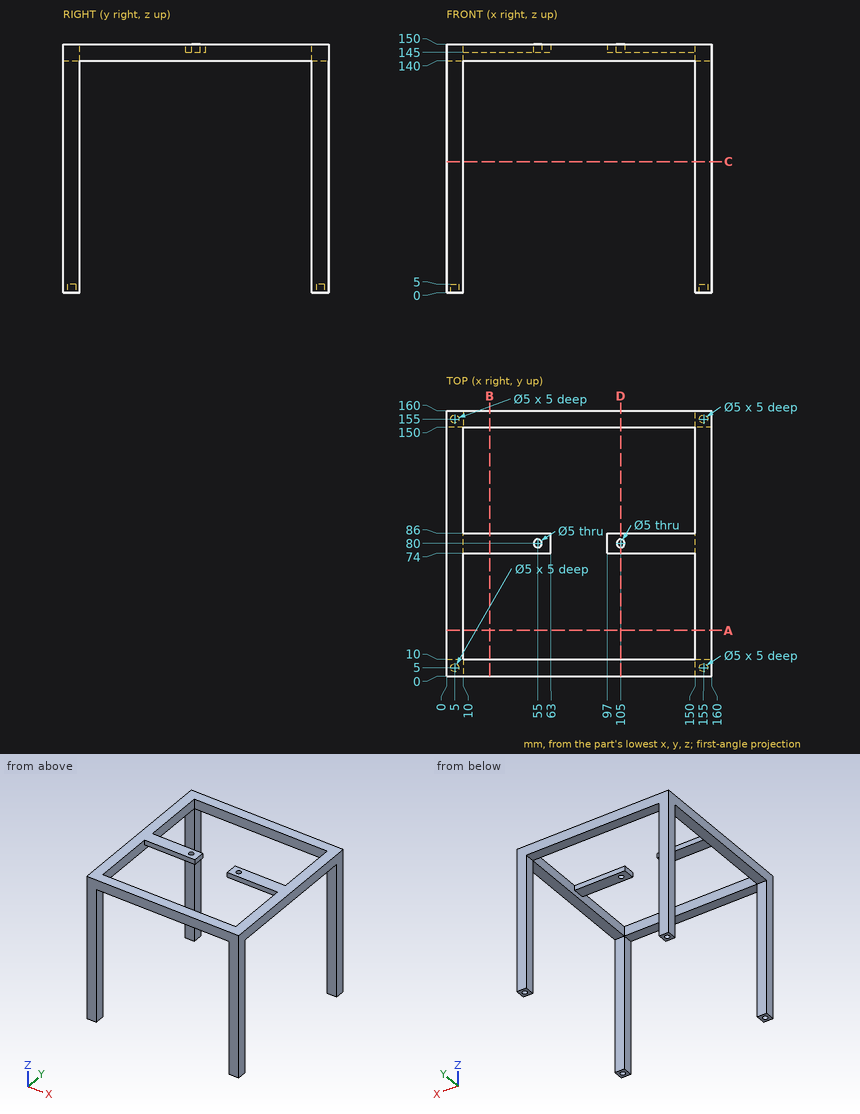
Design review of the part shown in the three views and the two pictorial views. Dimensions are in mm from the part's minimum x, y and z. Coordinates: 2 decimals unless noted, no trailing zeros. Loops run counter-clockwise (first coordinate to the right, second up) from the corner with the lowest first, then second, coordinate; pieces in that order, holes last. Notation, with made-up numbers: M 7.25,14.5 L 29.25,14.5 A12 cw 29.25,19.5 Z; hole C -6.75,-26.5 d6. An arc over 180 degrees is marked long. Put each result on its own line as item: value. Start each with the question number.
Q1. Wall thickness on line 1 (X direction, y = 5, z = 3.5); line 2 (X direction, y = 80, z = 148.05): over which ranges is each line inside the solid? List them lowest first.
Q2. Add section A-A (y = 27.5). Write out the cut boundary in (x, z).
Q3. Clearance check with flat-ended pins moving along their axes: pin 1 (10 mm diameter, centred on x = 16.5, z = 37, fed in from +Y); pin 2 (4.5 mm diameter, centred on x = 155, y = 155, fed in from -Z); pin 3 (5 mm diameter, centred on x = 154.5, y = 57.5, fed in from -Z). State where each tip first meets the part, or that it passes through.
Q4. Add section C-C (z = 79). Write out the cut boundary in (x, y), and give its area (3 significant figures).
Q5. Add section B-B (x = 26). Write out the cut boundary in (y, z).
Q6. Add section D-D (x = 105). Write out the cut boundary in (y, z), and give its area (3 significant figures).
Answers:
1. line 1: x = 0 to 2.5, 7.5 to 10, 150 to 152.5, 157.5 to 160
1. line 2: x = 0 to 52.5, 57.5 to 63, 97 to 102.5, 107.5 to 160
2. outline: M 0,140 L 10,140 L 10,150 L 0,150 Z; M 150,140 L 160,140 L 160,150 L 150,150 Z
3. pin 1: passes through
3. pin 2: stops at z = 5
3. pin 3: stops at z = 140
4. outline: M 0,0 L 10,0 L 10,10 L 0,10 Z; M 0,150 L 10,150 L 10,160 L 0,160 Z; M 150,0 L 160,0 L 160,10 L 150,10 Z; M 150,150 L 160,150 L 160,160 L 150,160 Z
4. area: 400 mm^2
5. outline: M 0,140 L 10,140 L 10,150 L 0,150 Z; M 74,145 L 86,145 L 86,150 L 74,150 Z; M 150,140 L 160,140 L 160,150 L 150,150 Z
6. outline: M 0,140 L 10,140 L 10,150 L 0,150 Z; M 74,145 L 77.5,145 L 77.5,150 L 74,150 Z; M 82.5,145 L 86,145 L 86,150 L 82.5,150 Z; M 150,140 L 160,140 L 160,150 L 150,150 Z
6. area: 235 mm^2
